Work out the finished part from the listing and answer in its coordinate system (mm). Round coordinates to 2 decimals unless told otherwise and drop trailing zeros. Order: outer loops, then holes, each group sorted by start corner. A loop starts at its lowest first (then second) coordinate and runs counter-clockwise, first axis right, second up. Notation, with made-up numbers: (35.5, 61.25) - (83.5, 61.25) arc R27 cw to (83.5, 89.25) - close; hole circle Ø11 at (32.5, 11). An arc over 180 degrees is marked (long way). Use one line per item in the form item = value. Start each with the question number.
Q1. The part is cut by section A-A on x = -22.5. Determine the outline of the cut face in (y, z), plus the area to 3 significant figures.
Q2. The part is cut by section C-C on y = 82. Determine the outline of the cut face in (x, z).
Q3. The part is cut by section B-B on x = -47. Determine the outline of the cut face in (y, z).
Q4. Find the intervals of material crossed by line 1 (X direction, y = 37.5, z = 5.5); line 2 (Y direction, x = -9, z = 5.5); line 3 (Y direction, x = -22, z = 10.25), in increasing order. Write a range as [from, to].
Q5. The part is cut by section D-D on x = -141.5. Determine the outline of the cut face in (y, z), plus the area to 3 significant figures.
from build123d import *

# Parameters (mm, degrees)
SKETCH1_W           = 152.4
SKETCH1_H           = 152.4
BOSS_EXTRUDE1_DEPTH = 12.7
SKETCH2_W           = 12.7
SKETCH2_H           = 127
CUT_EXTRUDE1_DEPTH  = 12.7
SKETCH3_W           = 7.62
SKETCH3_H           = 7.62
CUT_EXTRUDE2_DEPTH  = 25.4
SKETCH4_W           = 7.62
SKETCH4_H           = 7.62
CUT_EXTRUDE3_DEPTH  = 25.4
SKETCH5_W           = 7.62
SKETCH5_H           = 7.62
CUT_EXTRUDE4_DEPTH  = 25.4


with BuildPart() as part:
    # Sketch1 → Boss-Extrude1 (new body)
    with BuildSketch(Plane.XY):
        with Locations((-76.2, 76.2)):
            Rectangle(SKETCH1_W, SKETCH1_H)
    extrude(amount=BOSS_EXTRUDE1_DEPTH)

    # Sketch2 → Cut-Extrude1 (cut)
    with BuildSketch(Plane.XY.offset(12.7)):
        with Locations((-133.35, 76.2)):
            Rectangle(SKETCH2_W, SKETCH2_H)
        with Locations((-19.05, 76.2)):
            Rectangle(SKETCH2_W, SKETCH2_H)
        with Locations((-44.45, 76.2)):
            Rectangle(SKETCH2_W, SKETCH2_H)
        with Locations((-107.95, 76.2)):
            Rectangle(SKETCH2_W, SKETCH2_H)
        with Locations((-82.55, 76.2)):
            Rectangle(SKETCH2_W, SKETCH2_H)
        with Locations((-69.85, 76.2)):
            Rectangle(SKETCH2_W, SKETCH2_H)
    extrude(amount=-CUT_EXTRUDE1_DEPTH, mode=Mode.SUBTRACT)

    # Sketch3 → Cut-Extrude2 (cut)
    with BuildSketch(Plane(origin=(0, 0, 0), x_dir=(0, 0, -1), z_dir=(1, 0, 0))):
        with Locations((-6.35, 146.05)):
            Rectangle(SKETCH3_W, SKETCH3_H)
    extrude(amount=-CUT_EXTRUDE2_DEPTH, mode=Mode.SUBTRACT)

    # Sketch4 → Cut-Extrude3 (cut)
    with BuildSketch(Plane.ZY.offset(152.4)):
        with Locations((6.35, 146.05)):
            Rectangle(SKETCH4_W, SKETCH4_H)
    extrude(amount=-CUT_EXTRUDE3_DEPTH, mode=Mode.SUBTRACT)

    # Sketch5 → Cut-Extrude4 (cut)
    with BuildSketch(Plane.XZ):
        with Locations((-6.35, 6.35)):
            Rectangle(SKETCH5_W, SKETCH5_H)
    extrude(amount=-CUT_EXTRUDE4_DEPTH, mode=Mode.SUBTRACT)


solid = part.part
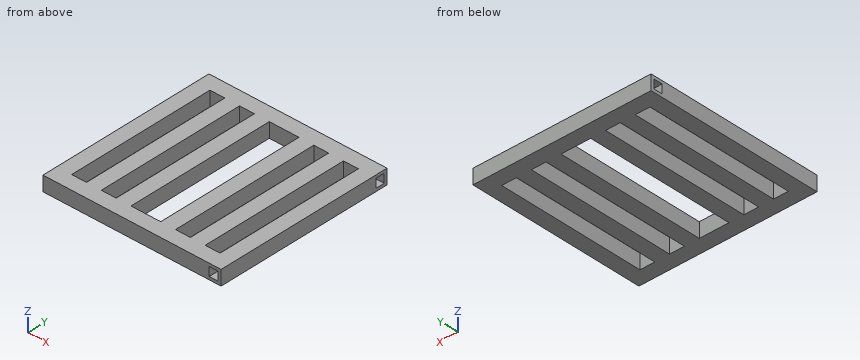
Found:
q1.outline = (0, 0) - (12.7, 0) - (12.7, 12.7) - (0, 12.7) - close; (139.7, 0) - (152.4, 0) - (152.4, 12.7) - (139.7, 12.7) - close; hole (142.24, 2.54) - (149.86, 2.54) - (149.86, 10.16) - (142.24, 10.16) - close
q1.area = 265 mm²
q2.outline = (-152.4, 0) - (-139.7, 0) - (-139.7, 12.7) - (-152.4, 12.7) - close; (-127, 0) - (-114.3, 0) - (-114.3, 12.7) - (-127, 12.7) - close; (-101.6, 0) - (-88.9, 0) - (-88.9, 12.7) - (-101.6, 12.7) - close; (-63.5, 0) - (-50.8, 0) - (-50.8, 12.7) - (-63.5, 12.7) - close; (-38.1, 0) - (-25.4, 0) - (-25.4, 12.7) - (-38.1, 12.7) - close; (-12.7, 0) - (0, 0) - (0, 12.7) - (-12.7, 12.7) - close
q3.outline = (0, 0) - (12.7, 0) - (12.7, 12.7) - (0, 12.7) - close; (139.7, 0) - (152.4, 0) - (152.4, 12.7) - (139.7, 12.7) - close
q4.line_1 = [-152.4, -139.7], [-127, -114.3], [-101.6, -88.9], [-63.5, -50.8], [-38.1, -25.4], [-12.7, 0]
q4.line_2 = [25.4, 142.24], [149.86, 152.4]
q4.line_3 = [0, 12.7], [139.7, 152.4]
q5.outline = (0, 0) - (152.4, 0) - (152.4, 12.7) - (0, 12.7) - close; hole (142.24, 2.54) - (149.86, 2.54) - (149.86, 10.16) - (142.24, 10.16) - close
q5.area = 1,880 mm²
